from build123d import *

# Parameters (mm, degrees)
SKETCH1_W           = 24
SKETCH1_H           = 50
BOSS_EXTRUDE1_DEPTH = 9.42
SKETCH2_W           = 6
SKETCH2_H           = 40
SKETCH2_W_2         = 9
SKETCH2_H_2         = 10
SKETCH2_W_3         = 5.4
BOSS_EXTRUDE2_DEPTH = 8
FILLET1_R           = 3
SKETCH4_R           = 1.625
CUT_EXTRUDE2_DEPTH  = 46.248827609
CUT_EXTRUDE3_DEPTH  = 2
SKETCH6_W           = 2
SKETCH6_H           = 40
CUT_EXTRUDE4_DEPTH  = 1
SKETCH7_R           = 1.125
CUT_EXTRUDE5_DEPTH  = 12
SKETCH9_R           = 1.625
CUT_EXTRUDE6_DEPTH  = 33.748380113
FILLET2_R           = 1
BOSS_EXTRUDE3_DEPTH = 8
LPATTERN1_COUNT     = 5
LPATTERN1_PITCH     = 2


with BuildPart() as part:
    # Sketch1 → Boss-Extrude1 (new body)
    with BuildSketch(Plane(origin=(0, 0, 0), x_dir=(1, 0, 0), z_dir=(0, 1, 0))):
        Rectangle(SKETCH1_W, SKETCH1_H)
    extrude(amount=BOSS_EXTRUDE1_DEPTH)

    # Sketch2 → Boss-Extrude2 (add)
    with BuildSketch(Plane(origin=(0, 9.42, 0), x_dir=(1, 0, 0), z_dir=(0, 1, 0))):
        with Locations((-9, 5)):
            Rectangle(SKETCH2_W, SKETCH2_H)
        with Locations((0, -20)):
            Rectangle(SKETCH2_W_2, SKETCH2_H_2)
        with Locations((9.3, -20)):
            Rectangle(SKETCH2_W_3, SKETCH2_H_2)
    extrude(amount=BOSS_EXTRUDE2_DEPTH)

    # Fillet1
    fillet1_edges = [part.edges().sort_by_distance(p)[0] for p in [
        (-12, 13.42, 15),
        (-6, 13.42, 15),
    ]]
    fillet(fillet1_edges, radius=FILLET1_R - 0.0001)  # a hair under: the kernel refuses the full size

    # Sketch4 → Cut-Extrude2 (cut, through all)
    with BuildSketch(Plane(origin=(0, 0, 15), x_dir=(-1, 0, 0), z_dir=(0, 0, -1))):
        with Locations((0, 12.42)):
            Circle(SKETCH4_R)
    extrude(amount=-CUT_EXTRUDE2_DEPTH, mode=Mode.SUBTRACT)

    # Sketch5 → Cut-Extrude3 (cut)
    with BuildSketch(Plane(origin=(0, 0, 15), x_dir=(-1, 0, 0), z_dir=(0, 0, -1))):
        Polygon((-2.875, 14.079882024), (-2.875, 17.42), (2.875, 17.42), (2.875, 14.079882024), (2.875, 10.760117976), (0, 9.100235952), (-2.875, 10.760117976), align=None)
    extrude(amount=-CUT_EXTRUDE3_DEPTH, mode=Mode.SUBTRACT)

    # Sketch6 → Cut-Extrude4 (cut)
    with BuildSketch(Plane(origin=(0, 9.42, 0), x_dir=(1, 0, 0), z_dir=(0, 1, 0))):
        with Locations((0, 5)):
            Rectangle(SKETCH6_W, SKETCH6_H)
    extrude(amount=-CUT_EXTRUDE4_DEPTH, mode=Mode.SUBTRACT)

    # Sketch7 → Cut-Extrude5 (cut)
    with BuildSketch(Plane.ZY.offset(12)):
        with Locations((20, 4.93)):
            Circle(SKETCH7_R)
    extrude(amount=-CUT_EXTRUDE5_DEPTH, mode=Mode.SUBTRACT)

    # Sketch9 → Cut-Extrude6 (cut, through all)
    with BuildSketch(Plane.XZ):
        with Locations(Location((9, 22, 0), (0, 0, 270))):
            Circle(SKETCH9_R)
        with Locations(Location((9, -22, 0), (0, 0, 270))):
            Circle(SKETCH9_R)
        with Locations(Location((-9, -22, 0), (0, 0, 270))):
            Circle(SKETCH9_R)
        with Locations(Location((-9, 10, 0), (0, 0, 270))):
            Circle(SKETCH9_R)
    extrude(amount=-CUT_EXTRUDE6_DEPTH, mode=Mode.SUBTRACT)

    # Fillet2
    fillet2_edges = [part.edges().sort_by_distance(p)[0] for p in [
        (-6, 13.42, -25),
        (-4.5, 13.42, 25),
        (4.5, 13.42, 25),
        (12, 13.42, 15),
        (6.6, 13.42, 25),
        (-12, 8.71, -25),
        (12, 4.71, -25),
        (12, 8.71, 25),
        (-12, 4.71, 25),
    ]]
    fillet(fillet2_edges, radius=FILLET2_R)

    # Sketch10 → Boss-Extrude3 (add)
    with BuildSketch(Plane(origin=(0, 9.42, 0), x_dir=(1, 0, 0), z_dir=(0, 1, 0))):
        Polygon((4.5, -24), (4.5, -23), (5.25, -23.25), (5.25, -23.75), align=None)
        Polygon((6.6, -24), (6.6, -23), (5.85, -23.25), (5.85, -23.75), align=None)
    boss_extrude3 = extrude(amount=BOSS_EXTRUDE3_DEPTH)

    # LPattern1: Boss-Extrude3 ×5
    with Locations(*[(0, 0, -i * LPATTERN1_PITCH) for i in range(1, LPATTERN1_COUNT)]):
        add(boss_extrude3)


solid = part.part
The model under review builds one solid part; all positions refer to its coordinate system, in mm. A direction names the side the tool comes from. Round coordinates to 2 decimals unless told otherwise and drop trailing zeros. Write each loop counter-clockwise with the first axis right and the second up, starting at its lowest first coordinate (ties: lowest second). Pieces come first, ordered by that corner, then holes. Notation, with made-up numbers: M 22.25,42 L 67.25,42 A27 cw 67.25,81 Z; hole C 78.25,-21 d9. An arc over 180 degrees is marked long. Answer as CSV lines item,"result". Start each with the question number.
Q1. Consider section C-C, the plane x = -8.25. Give the boundary of the cut face in (y, z) (3 decimals), then the cut area to 3 significant figures.
Q2. Tool access review of faces 1 (the face through (-2.875, 14, 16)), 2 (the face through (-4.199, 13.476, 24.715)), 3 (the face through (4.199, 13.476, 24.715)): name each direction out of +Z, -Z, +X, -X, +Y, -Y from which nothing blocks a thin tool from reaching the whole face with its end or side.
Q3. Consider section D-D, the plane z = -22. Give the boundary of the cut face in (x, y) (3 decimals), then the cut area to 3 significant figures.
Q4. Clearance check with flat-ended pins moving along their axes: P1, Ø1.5, axis at x = -9, z = 19, coming from the +Y side; P2, Ø1.1, axis at y = 14, z = 18.5, coming from the -X side; P3, Ø0.6, axis at y = 15, z = 15.5, coming from the +X side. State where each tip first meets the part, or that it passes through.
Q5. Wall thickness on line 1 along X through (y, z) = (6.75, -22) (3 decimals); line 2 along X through (y, z) = (13.5, 10) (3 decimals); line 3 along Z through (x, y) = (-9.5, 1.25): over which ranges is each line inside the solid? List them lowest first.
Q6. Consider section A-A, the plane z = 10. Give the boundary of the cut face in (x, y) (3 decimals).
Q7. Consider section B-B, the plane y = 4.93. Give the boundary of the cut face in (x, z) (3 decimals), then the cut area to 3 significant figures.
Q8. The part is to be moulded in two halves that separate along Z. For faces 4 (the face through (6.6, 13.4, 18.5)), 5 (the face through (0.21, 14.03, 20.94)), 6 (the face through (-8.51, 8.59, -23.55)), 7 (the face through (11.715, 13.476, 15.301)), say which applies: +Z half, -Z half, draft (parallel to the pull), parting line (faces both ways), or undercut.
Result set:
1,outline,"M 0,-25 L 17.42,-25 L 17.42,-23.442 L 0,-23.442 Z; M 0,-20.558 L 17.42,-20.558 L 17.42,8.558 L 0,8.558 Z; M 0,11.442 L 17.42,11.442 L 17.42,14.905 L 9.42,14.905 L 9.42,25 L 0,25 Z; hole C 4.93,20 d2.25"
1,area,"686 mm²"
2,face 1,"-Z, +Y"
2,face 2,"+Z, -X, +Y"
2,face 3,"+Z, +Y"
3,outline,"M -12,0 L -10.625,0 L -10.625,17.42 L -12,17.42 Z; M -7.375,0 L 7.375,0 L 7.375,9.42 L 1,9.42 L 1,8.42 L -1,8.42 L -1,9.42 L -6,9.42 L -6,17.42 L -7.375,17.42 Z; M 10.625,0 L 12,0 L 12,9.42 L 10.625,9.42 Z"
3,area,"185 mm²"
4,P1,"stops at y = 9.42"
4,P2,"stops at x = -4.5"
4,P3,"stops at x = 11.98"
5,line 1,"x = -12 to -10.625, -7.375 to 7.375, 10.625 to 12"
5,line 2,"x = -12 to -10.625, -7.375 to -6"
5,line 3,"z = -25 to -23.55, -20.45 to 8.45, 11.55 to 25"
6,outline,"M -12,0 L -10.625,0 L -10.625,17.42 L -12,17.42 Z; M -7.375,0 L 12,0 L 12,9.42 L 1,9.42 L 1,8.42 L -1,8.42 L -1,9.42 L -6,9.42 L -6,17.42 L -7.375,17.42 Z"
7,outline,"M -12,-24 A1 ccw -11,-25 L 11,-25 A1 ccw 12,-24 L 12,24 A1 ccw 11,25 L -11,25 A1 ccw -12,24 L -12,21.125 L 0,21.125 L 0,18.875 L -12,18.875 Z; hole C -9,-22 d3.25; hole C -9,10 d3.25; hole C 9,-22 d3.25; hole C 9,22 d3.25"
7,area,"1,140 mm²"
8,face 4,"undercut"
8,face 5,"draft"
8,face 6,"undercut"
8,face 7,"-Z half"
